Can you work these out from the model? Positions are in its coordinate system, mm. A direction names the side the tool comes from. Coordinates: 2 decimals unless noted, no trailing zeros. Order: outer loops, then holes, each group sorted by start corner. A loop starts at its lowest first (then second) coordinate and runs counter-clockwise, first axis right, second up. Notation, with made-up numbers: (24.5, -38) -> (59.5, -38) arc R31 cw to (59.5, -4) -> close; hole circle Ø9 at (57, 6.5). An arc over 180 degrees is marked (long way). Write item = value, one per line.
```python
from build123d import *

# Parameters (mm, degrees)
DODANIE_WYCI_GNI_CIE2_DEPTH = 5
SZKIC3_OUTSIDE_W            = 55.734
SZKIC3_OUTSIDE_H            = 53.724
SZKIC3_OUTSIDE_R            = 6.495190528
WYTNIJ_WYCI_GNI_CIE2_DEPTH  = 10
WYTNIJ_WYCI_GNI_CIE2_DRAFT  = 60
SZKIC4_R                    = 4
DODANIE_WYCI_GNI_CIE3_DEPTH = 80
ZAOKR_GLENIE1_R             = 1
SFAZOWANIE1_SIZE            = 1


with BuildPart() as part:
    # Szkic1 → Dodanie-wyciągnięcie2 (new body)
    with BuildSketch(Plane.XY):
        Polygon((3.75, 6.495190528), (-3.75, 6.495190528), (-7.5, 0), (-3.75, -6.495190528), (3.75, -6.495190528), (7.5, 0), align=None)
    extrude(amount=DODANIE_WYCI_GNI_CIE2_DEPTH)


with BuildPart() as wytnij_wyci_gni_cie2_tool:
    # Szkic3 outside → Wytnij-wyciągnięcie2 (with draft: the straight prism first)
    with BuildSketch(Plane.XY):
        Rectangle(SZKIC3_OUTSIDE_W, SZKIC3_OUTSIDE_H)
        Circle(SZKIC3_OUTSIDE_R, mode=Mode.SUBTRACT)
    extrude(amount=WYTNIJ_WYCI_GNI_CIE2_DEPTH)
    # Wytnij-wyciągnięcie2: the draft: its side faces are tilted about the plane it starts from
    wytnij_wyci_gni_cie2_sides = [wytnij_wyci_gni_cie2_tool.faces().sort_by_distance(p)[0] for p in [
        (0, -26.862, 5),
        (27.867, 0, 5),
        (0, 26.862, 5),
        (-27.867, 0, 5),
        (-6.495190528, 0, 5),
    ]]
    draft(wytnij_wyci_gni_cie2_sides, Plane.XY, WYTNIJ_WYCI_GNI_CIE2_DRAFT)


with BuildPart() as part_1:
    add(part.part)

    # Wytnij-wyciągnięcie2: cut by wytnij_wyci_gni_cie2_tool
    add(wytnij_wyci_gni_cie2_tool.part, mode=Mode.SUBTRACT)

    # Szkic4 → Dodanie-wyciągnięcie3 (add)
    with BuildSketch(Plane.XY):
        Circle(SZKIC4_R)
    extrude(amount=-DODANIE_WYCI_GNI_CIE3_DEPTH)

    # Zaokrąglenie1
    zaokr_glenie1_edges = [part_1.edges().sort_by_distance(p)[0] for p in [
        (-4, 0, 0),
    ]]
    fillet(zaokr_glenie1_edges, radius=ZAOKR_GLENIE1_R)

    # Sfazowanie1
    sfazowanie1_edges = [part_1.edges().sort_by_distance(p)[0] for p in [
        (-4, 0, -80),
    ]]
    chamfer(sfazowanie1_edges, length=SFAZOWANIE1_SIZE)


solid = part_1.part
```
Item 1: For faces 1 (the conical face through (-3.353, 5.841, 0.138)), 2 (the flat face through (2, -5, 0)), which set-ups out of +Z, -Z, +X, -X, +Y, -Y let a thin tool reach every point of the face, with its end or its side?
A:
face_1 = -Z, -X, +Y
face_2 = -Z
Item 2: I want a section at A-A, the plane z = -67.5. Please give me the cut outline in (x, y), plus the area to 3 significant figures.
A:
outline = circle Ø8 at (0, 0)
area = 50.3 mm2
Item 3: I'm going to push flat-ended pins straight in: P1, Ø6, axis at x = -4.5, y = -4.5, coming from the -Z side; P2, Ø6, axis at y = 1, z = -43, coming from the +X side; P3, Ø6, axis at y = -5, z = -6, coming from the -X side. Where does each tip first touch, or does it pass through?
A:
P1 = -79.64
P2 = 4
P3 = -3.46
Item 4: If I drill on probe 1 along Z at (x, y) = (-5.5, -1.75); probe 2 along Y at (x, z) = (0, -17); probe 3 along Y at (x, z) = (-2, -14), over which ranges is the centre line in solid material (lowest first)?
A:
probe_1 = 0 to 5
probe_2 = -4 to 4
probe_3 = -3.46 to 3.46
